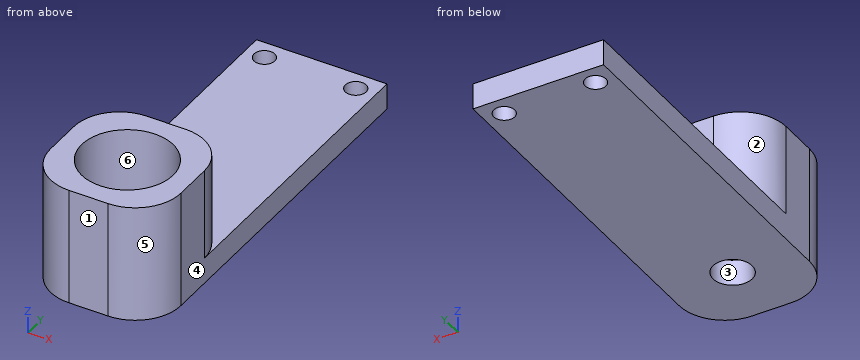
```python
from build123d import *

# Parameters (mm, degrees)
SKETCH1_W           = 10
SKETCH1_H           = 30
BOSS_EXTRUDE1_DEPTH = 2
SKETCH2_W           = 10
SKETCH2_H           = 10
SKETCH2_R           = 3.5
BOSS_EXTRUDE2_DEPTH = 7
SKETCH3_R           = 0.8
CUT_EXTRUDE1_DEPTH  = 2
FILLET1_R           = 3.5
SKETCH4_R           = 1.5
CUT_EXTRUDE2_DEPTH  = 2


with BuildPart() as part:
    # Sketch1 → Boss-Extrude1 (new body)
    with BuildSketch(Plane.XY):
        with Locations((-12.863567867, 6.68847884)):
            Rectangle(SKETCH1_W, SKETCH1_H)
    extrude(amount=BOSS_EXTRUDE1_DEPTH)

    # Sketch2 → Boss-Extrude2 (add)
    with BuildSketch(Plane.XY.offset(2)):
        with Locations((-12.863567867, -3.31152116)):
            Rectangle(SKETCH2_W, SKETCH2_H)
        with Locations((-12.863567867, -3.31152116)):
            Circle(SKETCH2_R, mode=Mode.SUBTRACT)
    extrude(amount=BOSS_EXTRUDE2_DEPTH)

    # Sketch3 → Cut-Extrude1 (cut)
    with BuildSketch(Plane.XY.offset(2)):
        with Locations((-16.363567867, 20.18847884)):
            Circle(SKETCH3_R)
        with Locations((-9.363567867, 20.18847884)):
            Circle(SKETCH3_R)
    extrude(amount=-CUT_EXTRUDE1_DEPTH, mode=Mode.SUBTRACT)

    # Fillet1
    fillet1_edges = [part.edges().sort_by_distance(p)[0] for p in [
        (-7.863567867, -8.31152116, 4.5),
        (-17.863567867, -8.31152116, 4.5),
        (-17.863567867, 1.68847884, 5.5),
        (-7.863567867, 1.68847884, 5.5),
    ]]
    fillet(fillet1_edges, radius=FILLET1_R)

    # Sketch4 → Cut-Extrude2 (cut)
    with BuildSketch(Plane.XY.offset(2)):
        with Locations((-12.863567867, -3.31152116)):
            Circle(SKETCH4_R)
    extrude(amount=-CUT_EXTRUDE2_DEPTH, mode=Mode.SUBTRACT)


solid = part.part
```
CAD build for the part. Positions are in the model's coordinates, mm. Face numbers are marked on the shaded views. A direction names the side the tool comes from. Coordinates: 2 decimals unless noted, no trailing zeros. Loops run counter-clockwise (first coordinate to the right, second up) from the corner with the lowest first, then second, coordinate; pieces in that order, holes last. Notation, with made-up numbers: (48.5, -33.75) - (73.5, -33.75) arc R7 cw to (73.5, -21.75) - close; hole circle Ø6 at (23, -18). An arc over 180 degrees is marked (long way). Use CSV: the item, a comma, the result in double quotes. Start each with the question number.
Q1. Cut at D-D, the plane y = 7.5. List the corners of the cut face in (x, z).
Q2. Probe probe 1 along Z at (x, y) = (-8.5, 2); probe 2 along Y at (x, z) = (-15.75, 3.25); probe 3 along Y at (x, z) = (-10, 1.5). List the from-to ranges inside material, lowest first. Write a range as from..to.
Q3. Cut at A-A, the plane x = -12.5. List the corners of the cut face in (y, z), then the cut area to 3 significant figures.
Q4. Two-plate mould, pull along Y, no slides. Class the marked faces 3, 4, 5 and 6: +Y half, -Y half, draft (parallel to the pull), parting line (faces both ways), or undercut.
Q5. Cut at B-B, the plane z = 1. List the corners of the cut face in (x, y).
Q6. 3-axis set-ups, long thin cutter, end or side, ignore diameter. For the marked faces 1 and 2: which of +Z, -Z, +X, -X, +Y, -Y reach the whole face in a straight line?
Q7. Drop flat-ended pins along their axis: P1, Ø2, axis at x = -10.5, y = 15, coming from the +Z side; P2, Ø2.5, axis at x = -13.5, z = 7, coming from the +Y side. Give the stop position or say it passes through.
Q8. Cut at C-C, the plane z = 6.5. List the corners of the cut face in (x, y), then the cut area to 3 significant figures.
Here are the results:
1,outline,"(-17.86, 0) - (-7.86, 0) - (-7.86, 2) - (-17.86, 2) - close"
2,probe 1,"0..2"
2,probe 2,"-8.03..-5.29, -1.33..1.4"
2,probe 3,"-8.03..19.7, 20.67..21.69"
3,outline,"(-8.31, 0) - (-4.77, 0) - (-4.77, 2) - (-6.79, 2) - (-6.79, 9) - (-8.31, 9) - close; (-1.86, 0) - (21.69, 0) - (21.69, 2) - (1.69, 2) - (1.69, 9) - (0.17, 9) - (0.17, 2) - (-1.86, 2) - close"
3,area,"75.4 mm2"
4,face 3,"undercut"
4,face 4,"draft"
4,face 5,"-Y half"
4,face 6,"undercut"
5,outline,"(-17.86, -4.81) arc R3.5 ccw to (-14.36, -8.31) - (-11.36, -8.31) arc R3.5 ccw to (-7.86, -4.81) - (-7.86, 21.69) - (-17.86, 21.69) - close; hole circle Ø1.6 at (-16.36, 20.19); hole circle Ø3 at (-12.86, -3.31); hole circle Ø1.6 at (-9.36, 20.19)"
6,face 1,"+Z, -Z, +X, -X, -Y"
6,face 2,"+Z, -X, +Y"
7,P1,"z = 2"
7,P2,"y = 1.69"
8,outline,"(-17.86, -4.81) arc R3.5 ccw to (-14.36, -8.31) - (-11.36, -8.31) arc R3.5 ccw to (-7.86, -4.81) - (-7.86, -1.81) arc R3.5 ccw to (-11.36, 1.69) - (-14.36, 1.69) arc R3.5 ccw to (-17.86, -1.81) - close; hole circle Ø7 at (-12.86, -3.31)"
8,area,"51.0 mm2"
